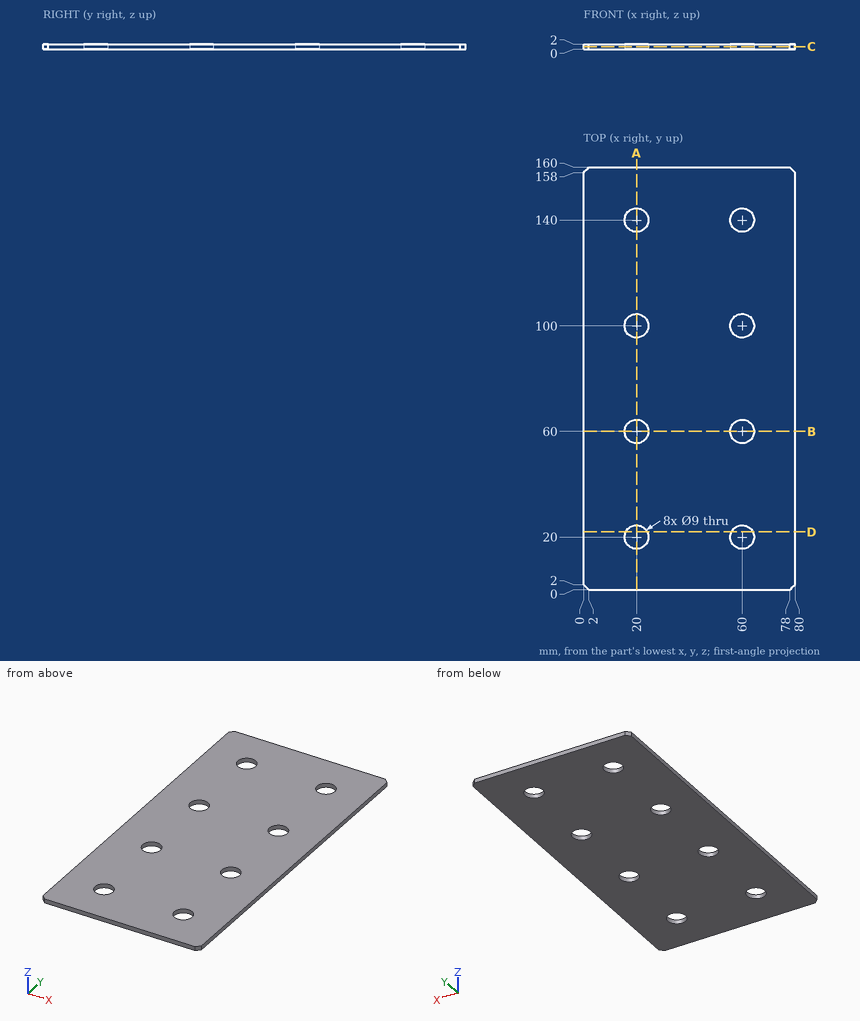
Drawing for the job (mm, zero at the part's lowest x, y, z). Round coordinates to 2 decimals unless told otherwise and drop trailing zeros. Loops run counter-clockwise (first coordinate to the right, second up) from the corner with the lowest first, then second, coordinate; pieces in that order, holes last. Notation, with made-up numbers: M -16.75,22.25 L -6.75,22.25 A13 ccw -6.75,38.25 Z; hole C 79.5,-40 d1. An arc over 180 degrees is marked long. Use a Markdown table: item, result. Add a question column.
(1) Cut at D-D (y = 22). Give the cut face in (x, z), and give its area (3 significant figures).
(2) Cut at A-A (x = 20). Give the cut face in (y, z), and give its area (3 significant figures).
(3) Flat gauge pin, fed straight in: pin 1 (5.5 mm diameter, centred on x = 60, y = 60, fed in from +Z). Where does the tip first touch, or does it go through?
(4) Cut at C-C (z = 1). State how many separate pieces and enclosed holes the cut face has, and give its area (3 significant figures).
(5) Drill centre lines: line 1 (Y direction, x = 60, z = 1.2); line 2 (Y direction, x = 18, z = 0.3); line 3 (X direction, y = 101, z = 0.6). Where is each one in solid material? Low to high.
(6) Cut at B-B (y = 60). Give the cut face in (x, z), and give its area (3 significant figures).
Geometry says:
| question | item | result |
|---|---|---|
| 1 | outline | M 0,0 L 15.97,0 L 15.97,2 L 0,2 Z; M 24.03,0 L 55.97,0 L 55.97,2 L 24.03,2 Z; M 64.03,0 L 80,0 L 80,2 L 64.03,2 Z |
| 1 | area | 128 mm² |
| 2 | outline | M 0,0 L 15.5,0 L 15.5,2 L 0,2 Z; M 24.5,0 L 55.5,0 L 55.5,2 L 24.5,2 Z; M 64.5,0 L 95.5,0 L 95.5,2 L 64.5,2 Z; M 104.5,0 L 135.5,0 L 135.5,2 L 104.5,2 Z; M 144.5,0 L 160,0 L 160,2 L 144.5,2 Z |
| 2 | area | 248 mm² |
| 3 | pin 1 | passes through |
| 4 | separate pieces | 1 |
| 4 | enclosed holes | 8 |
| 4 | area | 12,300 mm² |
| 5 | line 1 | y = 0 to 15.5, 24.5 to 55.5, 64.5 to 95.5, 104.5 to 135.5, 144.5 to 160 |
| 5 | line 2 | y = 0 to 15.97, 24.03 to 55.97, 64.03 to 95.97, 104.03 to 135.97, 144.03 to 160 |
| 5 | line 3 | x = 0 to 15.61, 24.39 to 55.61, 64.39 to 80 |
| 6 | outline | M 0,0 L 15.5,0 L 15.5,2 L 0,2 Z; M 24.5,0 L 55.5,0 L 55.5,2 L 24.5,2 Z; M 64.5,0 L 80,0 L 80,2 L 64.5,2 Z |
| 6 | area | 124 mm² |
